Autodesk Inventor part; units mm, degrees
ref_plane "YZ Plane" through (0, 0, 0) normal (1, 0, 0) x (0, 1, 0)
ref_plane "XZ Plane" through (0, 0, 0) normal (0, 1, 0) x (-1, 0, 0)
ref_plane "XY Plane" through (0, 0, 0) normal (0, 0, 1) x (1, 0, 0)
sketch "Sketch1" plane through (0, 0, 0) normal (0, 0, 1) x (1, 0, 0)
  line L0 (-30, 90) -> (30, 90)
  line L1 (30, 90) -> (30, -90)
  line L2 (30, -90) -> (-30, -90)
  line L3 (-30, -90) -> (-30, 90)
  point P0 (0, 0)
  point P1 (30, 0)
  point P2 (0, 90)
  dimension "d0" = 60
  dimension "d1" = 180
extrude "Extrusion1" add sketch "Sketch1" along normal blind 6
sketch "Sketch4" plane through (0, 0, 6) normal (0, 0, 1) x (1, 0, 0)
  line L0 (-15, 60) -> (15, 60)
  line L1 (15, 60) -> (15, -60)
  line L2 (15, -60) -> (-15, -60)
  line L3 (-15, -60) -> (-15, 60)
  line L4 (30, -90) -> (30, 90)
  line L5 (30, 90) -> (-30, 90)
  point P0 (0, 0)
  point P1 (0, 60)
  point P2 (15, 0)
  dimension "d20" = 15
  dimension "d21" = 30
extrude "Extrusion4" cut sketch "Sketch4" against normal through all
fillet "Fillet1" radius 5 8 edges at (-30, 90, 3) (30, 90, 3) (30, -90, 3) (-30, -90, 3) (-15, 60, 3) (15, 60, 3) (15, -60, 3) (-15, -60, 3)
chamfer "Chamfer2" distance 0.5 angle 45 32 edges at (0, 90, 6) (-28.5355, 88.5355, 6) (-30, 0, 6) (-28.5355, -88.5355, 6) (0, -90, 6) (28.5355, -88.5355, 6) (30, 0, 6) (28.5355, 88.5355, 6) (0, 90, 0) (-28.5355, 88.5355, 0) (-30, 0, 0) (-28.5355, -88.5355, 0) (0, -90, 0) (28.5355, -88.5355, 0) (30, 0, 0) (28.5355, 88.5355, 0) (-15, 0, 6) (-13.5355, 58.5355, 6) (0, 60, 6) (13.5355, 58.5355, 6) (15, 0, 6) (13.5355, -58.5355, 6) (0, -60, 6) (-13.5355, -58.5355, 6) (-15, 0, 0) (-13.5355, -58.5355, 0) (0, -60, 0) (13.5355, -58.5355, 0) (15, 0, 0) (13.5355, 58.5355, 0) (0, 60, 0) (-13.5355, 58.5355, 0)
equation "\"d0\" = width"
equation "\"d1\" = hight"
equation "\"hight\" = 180"
equation "\"width\" = 60"
properties part number "tc-top-bar" material "ABS Plastic"
Model file for the job. Use its own axes, mm. A direction names the side the tool comes from. Round coordinates to 2 decimals unless told otherwise and drop trailing zeros. Write each loop counter-clockwise with the first axis right and the second up, starting at its lowest first coordinate (ties: lowest second). Pieces come first, ordered by that corner, then holes. Notation, with made-up numbers: (13.25, -0.5) - (63.25, -0.5) arc R10 cw to (63.25, 15.5) - close; hole circle Ø10 at (22, 84.5). An arc over 180 degrees is marked (long way). Use CSV: the item, a comma, the result in double quotes. Start each with the question number.
Item 1: Tool access for faces 4 (the face through (13.596, -58.676, 5.642)), 5 (the face through (0, -60, 3)), 6 (the face through (-29, -88, 3)), 7 (the face through (13.596, 58.676, 0.358)), 8 (the face through (29, 88, 3)): list every direction of +Z, -Z, +X, -X, +Y, -Y with a clear straight run to the whole face (end or side of a thin tool).
Item 2: Drill centre lines: L1, parallel to Y at x = 5.5, z = 2.9; L2, parallel to X at y = -53, z = 5.1; L3, parallel to Y at x = -3, z = 5.7. Where is each one in solid material? Low to high. Write a range as [from, to].
Item 3: Pin check, flat tip, straight feed: P1, Ø10, axis at x = -1.5, y = 53.5, coming from the +Z side. Stop position of the tip, or through.
Item 4: Band-saw the part on A-A (z = 2.75). Write the cut outline in (x, y).
Item 5: Band-saw the part on B-B (y = 8.5). Write the cut outline in (x, z), and give its area (3 significant figures).
Item 6: Two-plate mould, pull along X, no slides. Class faces 1 (the face through (30, 1, 3)), 2 (the face through (-13, -59, 3)), 3 (the face through (19, 1, 0)): released by +X, released by -X, zero draft, split by the parting line, or undercut.
Checked values:
1,face 4,"+Z"
1,face 5,"+Z, -Z"
1,face 6,"+Z, -Z, -X, -Y"
1,face 7,"-Z"
1,face 8,"+Z, -Z, +X, +Y"
2,L1,"y = [-90, -60], [60, 90]"
2,L2,"x = [-30, -15], [15, 30]"
2,L3,"y = [-89.8, -60.2], [60.2, 89.8]"
3,P1,"passes through"
4,outline,"(-30, -85) arc R5 ccw to (-25, -90) - (25, -90) arc R5 ccw to (30, -85) - (30, 85) arc R5 ccw to (25, 90) - (-25, 90) arc R5 ccw to (-30, 85) - close; hole (-15, -55) arc R5 ccw to (-10, -60) - (10, -60) arc R5 ccw to (15, -55) - (15, 55) arc R5 ccw to (10, 60) - (-10, 60) arc R5 ccw to (-15, 55) - close"
5,outline,"(-30, 0.5) - (-29.5, 0) - (-15.5, 0) - (-15, 0.5) - (-15, 5.5) - (-15.5, 6) - (-29.5, 6) - (-30, 5.5) - close; (15, 0.5) - (15.5, 0) - (29.5, 0) - (30, 0.5) - (30, 5.5) - (29.5, 6) - (15.5, 6) - (15, 5.5) - close"
5,area,"179 mm²"
6,face 1,"released by +X"
6,face 2,"undercut"
6,face 3,"zero draft"
